from build123d import *

# Parameters (mm, degrees)
BOSS_EXTRUDE1_DEPTH = 2.5
SKETCH4_R           = 1.78
CUT_EXTRUDE1_DEPTH  = 1.5
FILLET1_R           = 1.5


with BuildPart() as part:
    # Sketch2 → Boss-Extrude1 (new body)
    with BuildSketch(Plane(origin=(0, 0, 0), x_dir=(1, 0, 0), z_dir=(0, 1, 0))):
        Polygon((-21.216153836, 11.741903429), (-21.216153836, 8.241903429), (-7.216153836, -0.958096571), (-0.216153836, -0.958096571), (7.783846164, 3.741903429), (7.783846164, 11.741903429), align=None)
    extrude(amount=BOSS_EXTRUDE1_DEPTH)

    # Sketch4 → Cut-Extrude1 (cut)
    with BuildSketch(Plane(origin=(0, 2.5, 0), x_dir=(1, 0, 0), z_dir=(0, 1, 0))):
        with Locations((-17.966153836, 8.241903429)):
            Circle(SKETCH4_R)
        with Locations((4.533846164, 8.241903429)):
            Circle(SKETCH4_R)
    extrude(amount=-CUT_EXTRUDE1_DEPTH, mode=Mode.SUBTRACT)

    # Fillet1
    fillet1_edges = [part.edges().sort_by_distance(p)[0] for p in [
        (7.783846164, 1.25, -11.741903429),
        (7.783846164, 1.25, -3.741903429),
        (-0.216153836, 1.25, 0.958096571),
        (-7.216153836, 1.25, 0.958096571),
        (-21.216153836, 1.25, -8.241903429),
        (-21.216153836, 1.25, -11.741903429),
        (7.783846164, 0, -7.741903429),
        (3.783846164, 0, -1.391903429),
        (-3.716153836, 0, 0.958096571),
        (-14.216153836, 0, -3.641903429),
        (-21.216153836, 0, -9.991903429),
        (-6.716153836, 0, -11.741903429),
    ]]
    fillet(fillet1_edges, radius=FILLET1_R)


solid = part.part
For this review, take the finished solid that the model builds, in its own axes (mm). Round coordinates to 2 decimals unless told otherwise and drop trailing zeros. Loops run counter-clockwise (first coordinate to the right, second up) from the corner with the lowest first, then second, coordinate; pieces in that order, holes last. Notation, with made-up numbers: (-5.75, 25) - (18.25, 25) arc R16 ccw to (18.25, 46) - close; hole circle Ø2 at (5.25, 61.25). An arc over 180 degrees is marked (long way). Use one line per item in the form item = value.
1) We need section A-A on y = 2.1. Write out the cut boundary in (x, z), then the cut area to 3 significant figures.
Solutions:
outline = (-21.22, -10.24) arc R1.5 ccw to (-19.72, -11.74) - (6.28, -11.74) arc R1.5 ccw to (7.78, -10.24) - (7.78, -4.6) arc R1.5 ccw to (7.04, -3.31) - (0.14, 0.75) arc R1.5 ccw to (-0.62, 0.96) - (-6.77, 0.96) arc R1.5 ccw to (-7.59, 0.71) - (-20.54, -7.8) arc R1.5 ccw to (-21.22, -9.05) - close; hole circle Ø3.56 at (-17.97, -8.24); hole circle Ø3.56 at (4.53, -8.24)
area = 264 mm2
2) Clearance check with flat-ended pins moving along their axes: P1, Ø4, axis at x = 5, z = -7.5, coming from the +Y side; P2, Ø1.8, axis at x = -17.5, z = -8.5, coming from the +Y side. State where each tip first meets the part, or that it passes through.
Solutions:
P1 = 2.5
P2 = 1
3) We need section C-C on y = 0.4. Write out the cut boundary in (x, z), then the cut area to 3 significant figures.
Solutions:
outline = (-20.74, -10.24) arc R1.02 ccw to (-19.72, -11.26) - (6.28, -11.26) arc R1.02 ccw to (7.3, -10.24) - (7.3, -4.6) arc R1.02 ccw to (6.8, -3.72) - (-0.11, 0.34) arc R1.02 ccw to (-0.62, 0.48) - (-6.77, 0.48) arc R1.02 ccw to (-7.33, 0.31) - (-20.28, -8.2) arc R1.02 ccw to (-20.74, -9.05) - close
area = 250 mm2
4) We need section B-B on z = -9.5. Write out the cut boundary in (x, y), then the cut area to 3 significant figures.
Solutions:
outline = (-21.22, 1.5) arc R1.5 ccw to (-19.72, 0) - (6.28, 0) arc R1.5 ccw to (7.78, 1.5) - (7.78, 2.5) - (5.79, 2.5) - (5.79, 1) - (3.27, 1) - (3.27, 2.5) - (-16.71, 2.5) - (-16.71, 1) - (-19.23, 1) - (-19.23, 2.5) - (-21.22, 2.5) - close
area = 64.0 mm2
5) Wall thickness on probe 1 along X at (y, z) = (1.9, -9.75); probe 2 along X at (y, z) = (1.55, -9); probe 3 along Z at (x, y) = (-18.25, 1.55): over which ranges is each line inside the solid? List them lowest first.
Solutions:
probe_1 = -21.22 to -18.91, -17.02 to 3.59, 5.48 to 7.78
probe_2 = -21.22 to -19.58, -16.36 to 2.92, 6.14 to 7.78
probe_3 = -11.74 to -10, -6.48 to -6.29
6) Mouldability with a two-part tool opening along X and no side actions: class faces 1 (the face through (-17.009, 1.76, -9.743)), 2 (the face through (-4, 0, -7)), 3 (the face through (4.302, 1.76, -10.007)), 4 (the face through (7.333, 2.007, -11.314)) as pulls with the +X half, pulls with the -X half, needs draft (parallel to the pull), parting line crosses it, or undercut.
Solutions:
face_1 = undercut
face_2 = needs draft
face_3 = undercut
face_4 = pulls with the +X half
